```python
from build123d import *

# Parameters (mm, degrees)
FILLET1_R = 5


with BuildPart() as part:
    # Sketch1 → Revolve1 (revolve)
    with BuildSketch(Plane.XY):
        with BuildLine():
            Line((-11.328734558, 50), (-15, 50))
            Line((-15, 50), (-15, 12.5))
            Line((-15, 12.5), (0, 12.5))
            Line((0, 12.5), (0, 40))
            ThreePointArc((0, 40), (-2.662495049, 40.590260942), (-4.826079992, 42.250438059))
            Line((-4.826079992, 42.250438059), (-11.328734558, 50))
        make_face()
    revolve1 = revolve(axis=Axis((-75.888260409, 0, 0), (1, 0, 0)))

    # Mirror1: Revolve1 across plane
    add(revolve1.mirror(Plane(origin=(0, 12.5, 0), x_dir=(0, 0, 1), z_dir=(-1, 0, 0))))

    # Fillet1
    fillet1_edges = [part.edges().sort_by_distance(p)[0] for p in [
        (11.328734558, -50, 0),
        (-11.328734558, -50, 0),
    ]]
    fillet(fillet1_edges, radius=FILLET1_R)


solid = part.part
```
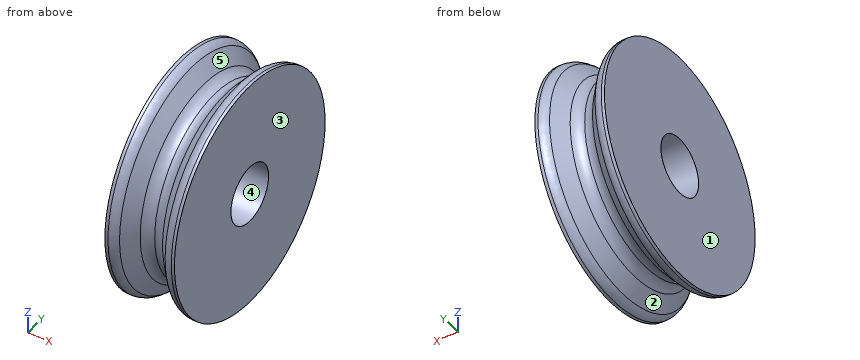
Read the model definition and answer for the solid it produces. Units are mm, in the model's axes. Face numbers are marked on the shaded views. A direction names the side the tool comes from. Give positions to 0.01 mm unless a question says otherwise; leave off trailing zeros. Order: outer loops, then holes, each group sorted by start corner. A loop starts at its lowest first (then second) coordinate and runs counter-clockwise, first axis right, second up.
(1) Given pin 1 (3 mm diameter, centred on x = -4, y = -8.5, fed in from -Z); pin 2 (4 mm diameter, centred on x = 3.5, y = -33.5, fed in from +Z); pin 3 (12 mm diameter, centred on x = 10, y = 25, fed in from +Z), each flat-ended and moving along its own axis, determine where each tip first touches the part or whether it passes through.
(2) For a pull along X with two mould halves and no side action, classify the marked faces 3, 4 and 5 as released by +X, released by -X, zero draft, split by the parting line, or undercut.
(3) Straight lines are drawn through the part: L1, parallel to X at y = 34, z = -31.5; L2, parallel to Z at x = 5.5, y = 0; L3, parallel to X at y = 40.5, z = 9. For each, find the intervals that lie inside material, in ascending order.
(4) Find section A-A (x = -1.5). Give the vertices of the cut face in (y, z).
(5) For the marked faces 1 and 2, determine the directions among +Z, -Z, +X, -X, +Y, -Y from which every point of the face is accessible in a straight line to the end or side of a thin tool.
Result sheet:
1. pin 1: stops at z = -42.23
1. pin 2: stops at z = 27.75
1. pin 3: stops at z = 45.88
2. face 3: released by +X
2. face 4: zero draft
2. face 5: undercut
3. L1: x = -15 to -8.27, 8.27 to 15
3. L2: z = -43.05 to -12.5, 12.5 to 43.05
3. L3: x = -15 to -4.07, 4.07 to 15
4. outline: circle Ø80.36 at (0, 0); hole circle Ø25 at (0, 0)
5. face 1: +Z, -Z, -X, +Y, -Y
5. face 2: none
